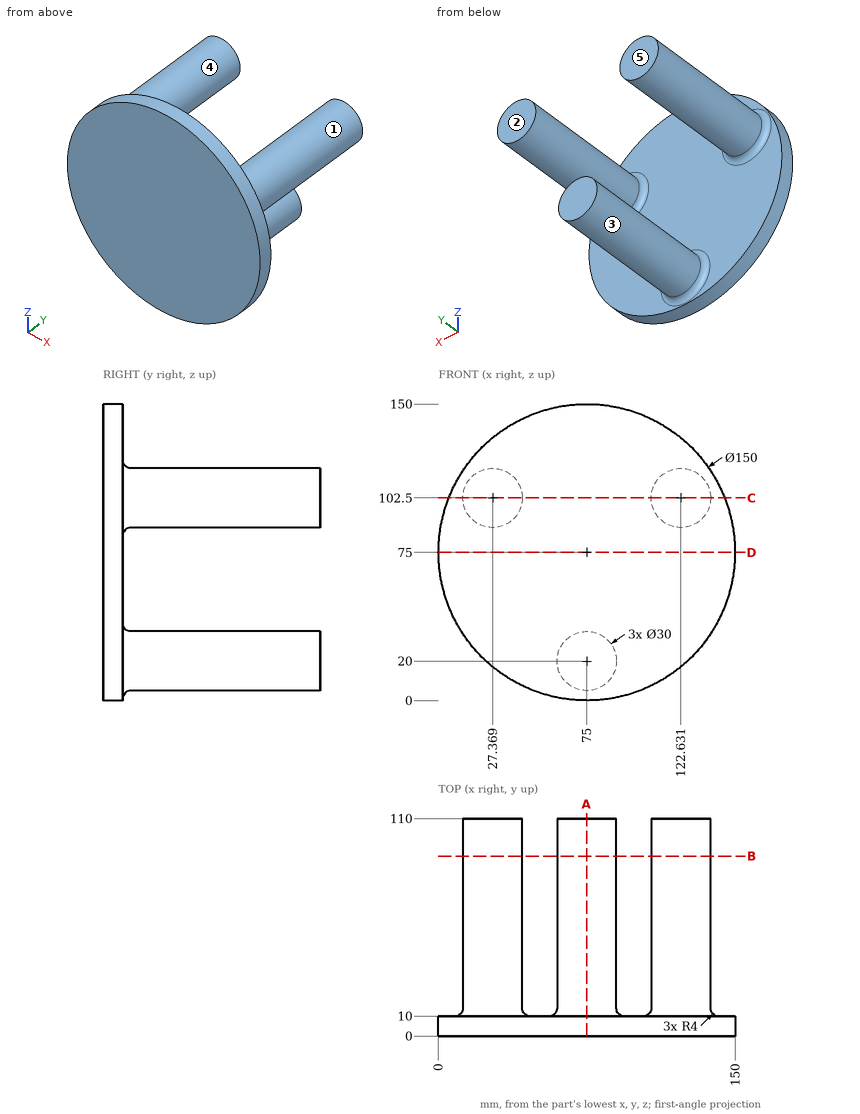
Geometry check sheet. Reference: drawing and pictorial views, mm from the part's lowest x, y, z. A direction names the side the tool comes from. Give positions to 0.01 mm unless a question says otherwise; leave off trailing zeros. Write each loop counter-clockwise with the first axis right and the second up, starting at its lowest first coordinate (ties: lowest second). Pieces come first, ordered by that corner, then holes.
Item 1: Cross-section at D-D (z = 75). Enter the section's corners in (x, y).
Item 2: Access from +Z, -Z, +X, -X, +Y, -Y to the whole of each face (thin tool, end or side, straight path). Record for the marked faces 1 and 2.
Item 3: Scan lines: L1, parallel to Y at x = 47, z = 116; L2, parallel to X at y = 17.5, z = 108 (1 decimal); L3, parallel to Z at x = 28.5, y = 16.5. Record each from-to range of solid material in increasing order.
Item 4: Cross-section at B-B (y = 91). Enter the section's corners in (x, z).
Item 5: Cross-section at C-C (z = 102.5). Enter the section's corners in (x, y).
Item 6: Draft check along X on the marked faces 3, 4 and 5. Enter one of: released by +X, released by -X, zero draft, split by the parting line, or undercut.
Item 7: Cross-section at A-A (x = 75). Enter the section's corners in (y, z), and give its area (3 significant figures).
Item 8: Gauge pin test, flat ends, axial feed: pin 1 (12 mm diameter, centred on x = 119, y = 29.5, fed in from +Z); pin 2 (2 mm diameter, centred on y = 71.5, z = 116.5, fed in from +X) (1 decimal); pin 3 (1.5 mm diameter, centred on x = 123, z = 30.5, fed in from +Y). Record the tip position at first contact, or that the pin passes through.
Report:
1. outline: (0, 0) - (150, 0) - (150, 10) - (0, 10) - close
2. face 1: +Y
2. face 2: +Z, -Z, +X, -X, +Y
3. L1: y = 0 to 10
3. L2: x = 13.4 to 41.3, 108.7 to 136.6
3. L3: z = 87.54 to 117.46
4. outline: circle Ø30 at (27.37, 102.5); circle Ø30 at (75, 20); circle Ø30 at (122.63, 102.5)
5. outline: (5.22, 0) - (144.78, 0) - (144.78, 10) - (141.63, 10) arc R4 cw to (137.63, 14) - (137.63, 110) - (107.63, 110) - (107.63, 14) arc R4 cw to (103.63, 10) - (46.37, 10) arc R4 cw to (42.37, 14) - (42.37, 110) - (12.37, 110) - (12.37, 14) arc R4 cw to (8.37, 10) - (5.22, 10) - close
6. face 3: split by the parting line
6. face 4: undercut
6. face 5: zero draft
7. outline: (0, 0) - (10, 0) - (10, 1) arc R4 cw to (14, 5) - (110, 5) - (110, 35) - (14, 35) arc R4 cw to (10, 39) - (10, 150) - (0, 150) - close
7. area: 4,510 mm2
8. pin 1: stops at z = 117.5
8. pin 2: stops at x = 130.1
8. pin 3: stops at y = 10
